```python
from build123d import *

# Parameters (mm, degrees)
SKETCH1_R                = 0.5
BOSS_EXTRUDE1_DEPTH      = 6.35
SKETCH2_W                = 3
SKETCH2_H                = 3
CUT_EXTRUDE1_DEPTH       = 6.35
FILLET1_R                = 2.54
M2_CLEARANCE_HOLE1_D     = 2.2
M2_CLEARANCE_HOLE1_DEPTH = 28.34894
M2_CLEARANCE_HOLE1_TIP   = 0.660946681
FILLET2_R                = 0.5
SKETCH6_W                = 1.5875
SKETCH6_H                = 1.5875
CUT_EXTRUDE2_DEPTH       = 21.329919454


with BuildPart() as part:
    # Sketch1 → Boss-Extrude1 (new body)
    with BuildSketch(Plane(origin=(0, 0, 0), x_dir=(0, 0, -1), z_dir=(1, 0, 0))):
        with BuildLine():
            Line((-18.783553311, 3.175), (18.783553311, 3.175))
            ThreePointArc((18.783553311, 3.175), (19.05, 0), (18.783553311, -3.175))
            Line((18.783553311, -3.175), (-18.783553311, -3.175))
            ThreePointArc((-18.783553311, -3.175), (-19.05, 0), (-18.783553311, 3.175))
        make_face()
        with Locations((6.35, 0)):
            Circle(SKETCH1_R, mode=Mode.SUBTRACT)
        with Locations((-6.35, 0)):
            Circle(SKETCH1_R, mode=Mode.SUBTRACT)
        Circle(SKETCH1_R, mode=Mode.SUBTRACT)
    extrude(amount=BOSS_EXTRUDE1_DEPTH)

    # Sketch2 → Cut-Extrude1 (cut)
    with BuildSketch(Plane(origin=(0, 3.175, 0), x_dir=(1, 0, 0), z_dir=(0, 1, 0))):
        with Locations((3.175, -15.5)):
            Rectangle(SKETCH2_W, SKETCH2_H)
        with Locations((3.175, 15.5)):
            Rectangle(SKETCH2_W, SKETCH2_H)
    extrude(amount=-CUT_EXTRUDE1_DEPTH, mode=Mode.SUBTRACT)

    # Fillet1
    fillet1_edges = [part.edges().sort_by_distance(p)[0] for p in [
        (0, 0, -5.85),
        (6.35, 0, -5.85),
        (0, 0, 6.85),
        (6.35, 0, 6.85),
    ]]
    fillet(fillet1_edges, radius=FILLET1_R)

    # M2 Clearance Hole1
    with Locations(Plane.XZ.offset(3.175)):
        with Locations((3.175, 9.525), (3.175, -9.525)):
            Hole(M2_CLEARANCE_HOLE1_D / 2, depth=M2_CLEARANCE_HOLE1_DEPTH)
            with Locations((0, 0, -(M2_CLEARANCE_HOLE1_DEPTH + M2_CLEARANCE_HOLE1_TIP / 2))):  # 118° drill point
                Cone(0, M2_CLEARANCE_HOLE1_D / 2, M2_CLEARANCE_HOLE1_TIP, mode=Mode.SUBTRACT)

    # Fillet2
    fillet2_edges = [part.edges().sort_by_distance(p)[0] for p in [
        (1.675, -3.175, 15.5),
        (3.175, -3.175, 14),
        (4.675, -3.175, 15.5),
        (3.175, -3.175, 17),
        (1.675, 3.175, 15.5),
        (3.175, 3.175, 17),
        (4.675, 3.175, 15.5),
        (3.175, 3.175, 14),
        (3.175, -3.175, -17),
        (4.675, -3.175, -15.5),
        (3.175, -3.175, -14),
        (1.675, -3.175, -15.5),
        (3.175, 3.175, -17),
        (1.675, 3.175, -15.5),
        (3.175, 3.175, -14),
        (4.675, 3.175, -15.5),
    ]]
    fillet(fillet2_edges, radius=FILLET2_R)

    # Sketch6 → Cut-Extrude2 (cut, through all)
    with BuildSketch(Plane.ZY):
        with Locations((0, -2.38125)):
            Rectangle(SKETCH6_W, SKETCH6_H)
        with Locations((0, 2.38125)):
            Rectangle(SKETCH6_W, SKETCH6_H)
    extrude(amount=-CUT_EXTRUDE2_DEPTH, mode=Mode.SUBTRACT)


solid = part.part
```
For this review, take the finished solid that the model builds, in its own axes (mm). A direction names the side the tool comes from. Coordinates: 2 decimals unless noted, no trailing zeros. Loops run counter-clockwise (first coordinate to the right, second up) from the corner with the lowest first, then second, coordinate; pieces in that order, holes last.
1. Add section D-D, the plane z = 15. Give the boundary of the cut face in (x, y) (3 decimals), then the cut area to 3 significant figures.
2. Mouldability with a two-part tool opening along X and no side actions: class faces 5 (the flat face through (6.35, 1, 0)), 6 (the flat face through (3, 0, -17)), 7 (the flat face through (3, 2, 0.794)) as +X half, -X half, draft (parallel to the pull), parting line (faces both ways), or undercut.
3. Insertion check: P1, Ø3.5, axis at y = 1.5, z = 15, coming from the -X side; P2, Ø1.3, axis at x = 1.5, y = -2.5, coming from the -Z side; P3, Ø0.5, axis at x = 2, z = -0.5, coming from the -Y side; P4, Ø2, axis at x = 4, y = 2.5, coming from the +Z side. Each pin has a flat end and moves straight along its axis. Give the tip position at first contact, or say it passes through.
4. Add section B-B, the plane y = 0. Count the separate pieces of the cut face and the enclosed holes in it, then the cut area to 3 significant figures.
5. Add section A-A, the plane z = 6.35. Give the boundary of the cut face in (x, y) (3 decimals), then the cut area to 3 significant figures.
6. For line 1 (X direction, y = 2.75, z = 15); line 2 (Y direction, x = 2, z = 0); line 3 (Y direction, x = 3.35, z = 6.35) (3 decimals), list the stretches that pass through material, from the lowest coordinate up.
7. For faces 1 (the flat face through (3, 2, -0.794)), 2 (the flat face through (3, -1.588, 0)), 3 (the cylindrical face through (3.13, -0.04, 19.05)), 4 (the flat face through (1.675, 0, -15)), list the 3-axis set-ups (+Z, -Z, +X, -X, +Y, -Y) from which the entire face can be reached by the end or side of a thin tool; tool diameter is ignored.
Result:
1. outline: (0, -3.175) - (1.175, -3.175) arc R0.5 ccw to (1.675, -2.675) - (1.675, 2.675) arc R0.5 ccw to (1.175, 3.175) - (0, 3.175) - close; (4.675, -2.675) arc R0.5 ccw to (5.175, -3.175) - (6.35, -3.175) - (6.35, 3.175) - (5.175, 3.175) arc R0.5 ccw to (4.675, 2.675) - close
1. area: 21.1 mm2
2. face 5: +X half
2. face 6: undercut
2. face 7: draft
3. P1: stops at x = 0
3. P2: stops at z = -18.96
3. P3: stops at y = -1.59
3. P4: stops at z = 18.99
4. separate pieces: 4
4. enclosed holes: 4
4. area: 186 mm2
5. outline: (0, -3.175) - (6.35, -3.175) - (6.35, -3.04) arc R2.54 ccw to (3.81, -0.5) - (2.54, -0.5) arc R2.54 ccw to (0, -3.04) - close; (0, 3.04) arc R2.54 ccw to (2.54, 0.5) - (3.81, 0.5) arc R2.54 ccw to (6.35, 3.04) - (6.35, 3.175) - (0, 3.175) - close
5. area: 28.4 mm2
6. line 1: x = 0 to 1.67, 4.68 to 6.35
6. line 2: y = -1.59 to -0.5, 0.5 to 1.59
6. line 3: y = -3.175 to -0.5, 0.5 to 3.175
7. face 1: +X, -X, +Y
7. face 2: +X, -X, -Y
7. face 3: +Z, +X, -X
7. face 4: +Y, -Y
